from build123d import *

# Parameters (mm, degrees)
SKETCH1_W           = 203.708
SKETCH1_H           = 256.54
BOSS_EXTRUDE1_DEPTH = 6.35
CUT_EXTRUDE1_REACH  = 326.339
SKETCH2_R           = 11.1125


with BuildPart() as part:
    # Sketch1 → Boss-Extrude1 (new body)
    with BuildSketch(Plane.XY):
        with Locations((81.646636302, 139.093604852)):
            Rectangle(SKETCH1_W, SKETCH1_H)
    extrude(amount=BOSS_EXTRUDE1_DEPTH)

    # Sketch2 → Cut-Extrude1 (cut, up to next)
    with BuildSketch(Plane(origin=(0, 0, 0), x_dir=(-1, 0, 0), z_dir=(0, 0, -1)), mode=Mode.PRIVATE) as cut_extrude1_sk1:
        with Locations((-145.400636302, 202.593604852)):
            Circle(SKETCH2_R)
    cut_extrude1_tool1 = extrude(cut_extrude1_sk1.sketch, amount=-CUT_EXTRUDE1_REACH, mode=Mode.PRIVATE) & part.part
    # Sketch2 → Cut-Extrude1 (cut, up to next)
    with BuildSketch(Plane(origin=(0, 0, 0), x_dir=(-1, 0, 0), z_dir=(0, 0, -1)), mode=Mode.PRIVATE) as cut_extrude1_sk2:
        with Locations((-145.400636302, 75.593604852)):
            Circle(SKETCH2_R)
    cut_extrude1_tool2 = extrude(cut_extrude1_sk2.sketch, amount=-CUT_EXTRUDE1_REACH, mode=Mode.PRIVATE) & part.part
    # Sketch2 → Cut-Extrude1 (cut, up to next)
    with BuildSketch(Plane(origin=(0, 0, 0), x_dir=(-1, 0, 0), z_dir=(0, 0, -1)), mode=Mode.PRIVATE) as cut_extrude1_sk3:
        with Locations((-17.892636302, 202.593604852)):
            Circle(SKETCH2_R)
    cut_extrude1_tool3 = extrude(cut_extrude1_sk3.sketch, amount=-CUT_EXTRUDE1_REACH, mode=Mode.PRIVATE) & part.part
    # Sketch2 → Cut-Extrude1 (cut, up to next)
    with BuildSketch(Plane(origin=(0, 0, 0), x_dir=(-1, 0, 0), z_dir=(0, 0, -1)), mode=Mode.PRIVATE) as cut_extrude1_sk4:
        with Locations((-17.892636302, 75.593604852)):
            Circle(SKETCH2_R)
    cut_extrude1_tool4 = extrude(cut_extrude1_sk4.sketch, amount=-CUT_EXTRUDE1_REACH, mode=Mode.PRIVATE) & part.part
    add(cut_extrude1_tool1.solids().sort_by_distance((145.400636, 202.593605, 0))[0], mode=Mode.SUBTRACT)
    add(cut_extrude1_tool2.solids().sort_by_distance((145.400636, 75.593605, 0))[0], mode=Mode.SUBTRACT)
    add(cut_extrude1_tool3.solids().sort_by_distance((17.892636, 202.593605, 0))[0], mode=Mode.SUBTRACT)
    add(cut_extrude1_tool4.solids().sort_by_distance((17.892636, 75.593605, 0))[0], mode=Mode.SUBTRACT)


solid = part.part
Check sheet for the modelled part. Datum: model origin and axes. Units: mm. Round coordinates to 2 decimals unless told otherwise and drop trailing zeros. Order: outer loops, then holes, each group sorted by start corner. A loop starts at its lowest first (then second) coordinate and runs counter-clockwise, first axis right, second up.
(1) Cross-section at A-A, the plane x = 143. Enter the section's corners in (y, z), and give its area (3 significant figures).
(2) Scan lines: probe 1 along Y at (x, z) = (24.5, 6); probe 2 along Y at (x, z) = (23.5, 0.75); probe 3 along X at (y, z) = (205.5, 3.5). Record each from-to range of solid material in increasing order.
(3) Cross-section at B-B, the plane z = 4.25. Enter the section's corners in (x, y) (1 decimal).
(4) Go/stop test with a flat-tipped pin: P1, Ø18, axis at x = 17.89, y = 75.59, coming from the +Z side. Record where the tip stops, or that it passes through.
(5) Cross-section at C-C, the plane x = 16.5. Enter the section's corners in (y, z), and give its area (3 significant figures).
(6) Draft check along X on faces 1 (the flat face through (80, 10.824, 3)), 2 (the flat face through (183.501, 137, 3)), 3 (the cylindrical face through (134.8, 78.93, 3.13)), 4 (the cylindrical face through (7.293, 78.931, 3.131)). Enter one of: pulls with the +X half, pulls with the -X half, needs draft (parallel to the pull), parting line crosses it, or undercut.
Check sheet entries:
1. outline: (10.82, 0) - (64.74, 0) - (64.74, 6.35) - (10.82, 6.35) - close; (86.44, 0) - (191.74, 0) - (191.74, 6.35) - (86.44, 6.35) - close; (213.44, 0) - (267.36, 0) - (267.36, 6.35) - (213.44, 6.35) - close
1. area: 1,350 mm2
2. probe 1: y = 10.82 to 66.66, 84.53 to 193.66, 211.53 to 267.36
2. probe 2: y = 10.82 to 66, 85.19 to 193, 212.19 to 267.36
2. probe 3: x = -20.21 to 7.17, 28.62 to 134.67, 156.13 to 183.5
3. outline: (-20.2, 10.8) - (183.5, 10.8) - (183.5, 267.4) - (-20.2, 267.4) - close; hole circle Ø22.2 at (17.9, 75.6); hole circle Ø22.2 at (17.9, 202.6); hole circle Ø22.2 at (145.4, 75.6); hole circle Ø22.2 at (145.4, 202.6)
4. P1: passes through
5. outline: (10.82, 0) - (64.57, 0) - (64.57, 6.35) - (10.82, 6.35) - close; (86.62, 0) - (191.57, 0) - (191.57, 6.35) - (86.62, 6.35) - close; (213.62, 0) - (267.36, 0) - (267.36, 6.35) - (213.62, 6.35) - close
5. area: 1,350 mm2
6. face 1: needs draft
6. face 2: pulls with the +X half
6. face 3: undercut
6. face 4: undercut
